Autodesk Inventor part; units mm, degrees
ref_plane "YZ Plane" through (0, 0, 0) normal (1, 0, 0) x (0, 1, 0)
ref_plane "XZ Plane" through (0, 0, 0) normal (0, 1, 0) x (-1, 0, 0)
ref_plane "XY Plane" through (0, 0, 0) normal (0, 0, 1) x (1, 0, 0)
sketch "草圖1" plane through (0, 0, 0) normal (0, 0, 1) x (1, 0, 0)
  line L0 (-0.4423, 6) -> (-1.3723, 6)
  line L1 (-0.4423, 0) -> (-0.4423, 6) construction
  line L2 (-1.3723, 0) -> (0, 0) construction
  line L3 (-1.3723, 0) -> (-1.3723, 6) construction
  line L4 (-1.4073, -0.0008) -> (-1.4073, -7.2)
  line L5 (-1.4073, -7.2) -> (0.129, -7.2)
  line L6 (0.129, -7.2) -> (0.129, -1.2)
  line L7 (11.0577, 0) -> (8.0577, 0)
  line L8 (0.129, -1.2) -> (12.5577, -1.2)
  line L9 (12.5577, -1.2) -> (12.5577, 0)
  line L10 (12.5577, 0) -> (-0.4073, 0)
  line L11 (-0.4073, 0) -> (-0.4073, 3)
  line L12 (-0.4073, 3) -> (-1.4073, 3)
  line L13 (-1.4073, 3) -> (-1.4073, -0.0008)
  point P0 (-0.9073, 3)
  point P1 (9.5577, 0)
  dimension "d0" = 1
  dimension "d1" = 0.465
  dimension "d2" = 0.93
  dimension "d3" = 1.2
  dimension "d5" = 6
  dimension "d6" = 1.5
  dimension "d7" = 3
extrude "擠出1" add sketch "草圖1" along normal blind 6
sketch "草圖2" plane through (0.129, -1.2, 0) normal (0, -1, 0) x (1, 0, 0)
  circle A0 centre (9.4287, 2.9292) radius 1.5
  point P0 (-0.129, 0)
extrude "擠出2" cut sketch "草圖2" against normal blind 4.2
fillet "圓角1" radius 3 2 edges at (12.5577, -0.6, 6) (12.5577, -0.6, 0)
properties part number "j1 endstop blocker"
Here's how the part is built. I have some questions about the finished solid (model axes, mm). A direction names the side the tool comes from. Coordinates: 2 decimals unless noted, no trailing zeros. Order: outer loops, then holes, each group sorted by start corner. A loop starts at its lowest first (then second) coordinate and runs counter-clockwise, first axis right, second up. Notation, with made-up numbers: (-18, 46.25) - (9, 46.25) arc R15 ccw to (9, 71.25) - close; hole circle Ø8 at (56, 40.5). An arc over 180 degrees is marked (long way). One line per question, with ' | ' between items.
(1) Suppose I cut it at B-B on x = 10.25. List the corners of the cut face in (y, z) for me, and give its area (3 significant figures).
Report:
outline: (-1.2, 0.08) - (0, 0.08) - (0, 1.6) - (-1.2, 1.6) - close; (-1.2, 4.26) - (0, 4.26) - (0, 5.92) - (-1.2, 5.92) - close | area: 3.81 mm2
(2) If we mould it in two halves opening along X, with no side actions, what happens to faces 1 (the cylindrical face through (10.94, -0.61, 2.35)), 2 (the flat face through (0.129, -4, 3)), 3 (the flat face through (2, -1, 6))? For each: pulls with the +X half, pulls with the -X half, needs draft (parallel to the pull), parting line crosses it, or undercut.
Report:
face 1: undercut | face 2: pulls with the +X half | face 3: needs draft
(3) If I drill on L1, parallel to X at y = 0.5, z = 1.1; L2, parallel to X at y = -5.5, z = 1.35; L3, parallel to Y at x = 5, z = 4.6, over which ranges is the centre line in solid material (lowest first)?
Report:
L1: x = -1.41 to -0.41 | L2: x = -1.41 to 0.13 | L3: y = -1.2 to 0
(4) Suppose I cut it at A-A on z = 3.95. List the corners of the cut face in (x, y) for me, and give its area (3 significant figures).
Report:
outline: (-1.41, -7.2) - (0.13, -7.2) - (0.13, -1.2) - (8.46, -1.2) - (8.46, 0) - (-0.41, 0) - (-0.41, 3) - (-1.41, 3) - close; (10.66, -1.2) - (12.4, -1.2) - (12.4, 0) - (10.66, 0) - close | area: 26.2 mm2
(5) Suppose I cut it at D-D on y = 0.25. List the corners of the cut face in (x, z) for me.
Report:
outline: (-1.41, 0) - (-0.41, 0) - (-0.41, 6) - (-1.41, 6) - close
(6) For faces 4 (the flat face through (-0.407, 1, 3)), 5 (the flat face through (2, -1, 0)), 6 (the flat face through (6, -1.2, 3)), which set-ups out of +Z, -Z, +X, -X, +Y, -Y let a thin tool reach every point of the face, with its end or its side?
Report:
face 4: +Z, -Z, +X, +Y | face 5: -Z, +X, -X, +Y, -Y | face 6: +Z, -Z, +X, -Y
(7) Will these pins go through, and if not, where does the flat tip stop? pin 1 (1.5 mm diameter, centred on y = 2, z = 2.5, fed in from +X); pin 2 (1 mm diameter, centred on y = -1.5, z = 3.5, fed in from +X); pin 3 (3 mm diameter, centred on x = 4, z = 2, fed in from +Y).
Report:
pin 1: stops at x = -0.41 | pin 2: stops at x = 12.56 | pin 3: stops at y = 0
(8) Suppose I cut it at C-C on z = 4.7. List the corners of the cut face in (x, y) for me.
Report:
outline: (-1.41, -7.2) - (0.13, -7.2) - (0.13, -1.2) - (12.03, -1.2) - (12.03, 0) - (-0.41, 0) - (-0.41, 3) - (-1.41, 3) - close
